Geometry: final body of the model. Coordinates: model frame, mm. Face numbers are marked on the shaded views. A direction names the side the tool comes from. Coordinates: 2 decimals unless noted, no trailing zeros. Loops run counter-clockwise (first coordinate to the right, second up) from the corner with the lowest first, then second, coordinate; pieces in that order, holes last. Notation, with made-up numbers: (-22.5, 82.25) -> (-14.5, 82.25) arc R14 cw to (-14.5, 92.25) -> close; hole circle Ø1 at (57, -33.75). An arc over 180 degrees is marked (long way). One line per item, written item: value. Start each with the question number.
Item 1: Section query A-A on x = 0. Return loops of the section in (y, z).
Item 2: Set-up query: the marked faces 3 and 4. Return all of +Z, -Z, +X, -X, +Y, -Y with unobstructed straight access to the full face (end or side cutting, diameter ignored); none if empty.
Item 3: Mould query, pull axis X, two halves, no side actions, for the marked faces 1 and 2. Classes: +X half, -X half, draft (parallel to the pull), parting line (faces both ways), or undercut.
Item 4: Section query D-D on z = 4.86. Return loops of the section in (x, y).
Item 5: Section query B-B on z = 0. Return loops of the section in (x, y), then the cut area to 3 significant figures.
Item 6: Contact query for a flat-ended pin moving along its axis: pin 1 Ø2.5 at (x, z) = (6, 4.86) entering from -Y. Output: stop coordinate, or through.
Item 7: Section query C-C on y = 0.7. Return loops of the section in (x, z), then the cut area to 3 significant figures.
Item 8: Ray query, probe 1 along Z at (x, y) = (6, 0.65); probe 2 along X at (y, z) = (0.2, 4.86); probe 3 along X at (y, z) = (0.4, -5.5). Return the intervals inside material, ascending. Write a range as from..to.
Autodesk Inventor part; units mm, degrees
ref_plane "YZ Plane" through (0, 0, 0) normal (1, 0, 0) x (0, 1, 0)
ref_plane "XZ Plane" through (0, 0, 0) normal (0, 1, 0) x (-1, 0, 0)
ref_plane "XY Plane" through (0, 0, 0) normal (0, 0, 1) x (1, 0, 0)
sketch "Sketch1" plane through (0, 0, 0) normal (0, 1, 0) x (-1, 0, 0)
  line L0 (-7.5, 6.36) -> (7.5, 6.36)
  line L1 (7.5, 6.36) -> (7.5, -6.36)
  line L2 (7.5, -6.36) -> (-7.5, -6.36)
  line L3 (-7.5, -6.36) -> (-7.5, 6.36)
  line L4 (-7.5, 6.36) -> (7.5, -6.36) construction
  line L5 (7.5, 6.36) -> (-7.5, -6.36) construction
  point P0 (0, 0)
  dimension "d0" = 12.72
  dimension "d1" = 15
extrude "Extrusion1" add sketch "Sketch1" along normal blind 1
sketch "Sketch2" plane through (0, 1, 0) normal (0, 1, 0) x (1, 0, 0)
  circle A0 centre (0, 0) radius 4
  dimension "d4" = 8
extrude "Extrusion2" cut sketch "Sketch2" against normal up to surface (1 mm away)
sketch "Sketch3" plane through (0, 0, 0) normal (0, -1, 0) x (1, 0, 0)
  circle A0 centre (0, 0) radius 4
  circle A1 centre (0, 0) radius 6
  dimension "d7" = 12
  dimension "d8" = 8
extrude "Extrusion3" add sketch "Sketch3" along normal blind 0.46
sketch "Sketch4" plane through (0, 1, 0) normal (0, 1, 0) x (1, 0, 0)
  point P0 (0, 0)
sketch "Sketch5" plane through (0, 1, 0) normal (0, 1, 0) x (1, 0, 0)
  circle A0 centre (-6, -4.86) radius 0.8
  line L0 (-7.5, 6.36) -> (-7.5, -6.36)
  line L1 (-7.5, 0) -> (7.5, 0) construction
  line L2 (7.5, -6.36) -> (7.5, 6.36)
  line L3 (-7.5, -6.36) -> (7.5, -6.36)
  line L4 (0, -6.36) -> (0, 6.36) construction
  line L5 (7.5, 6.36) -> (-7.5, 6.36)
  circle A1 centre (-6, 4.86) radius 0.8
  line L6 (0, 6.36) -> (0, -6.36) construction
  circle A2 centre (6, -4.86) radius 0.8
  circle A3 centre (6, 4.86) radius 0.8
  point P0 (0, 0)
  dimension "d11" = 1.5
  dimension "d12" = 1.6
  dimension "d13" = 1.5
extrude "Extrusion4" cut sketch "Sketch5" against normal up to surface (1 mm away) contours A0 | A1 | A2 | A3
properties part number "PinholeFlexFixture" material "Acetal Resin, Black"
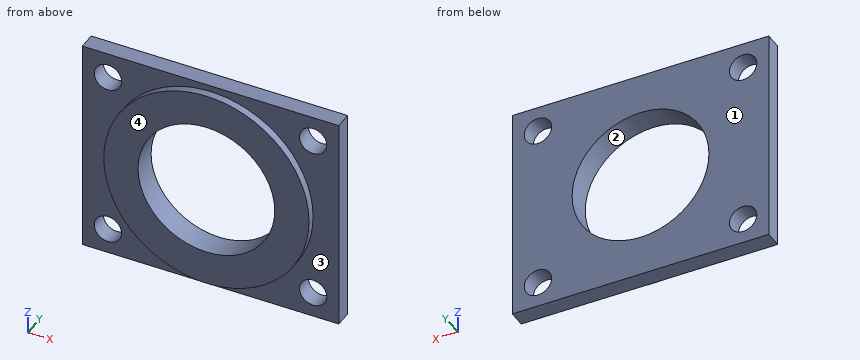
Reply:
1. outline: (-0.46, -6) -> (0, -6) -> (0, -6.36) -> (1, -6.36) -> (1, -4) -> (-0.46, -4) -> close; (-0.46, 4) -> (1, 4) -> (1, 6.36) -> (0, 6.36) -> (0, 6) -> (-0.46, 6) -> close
2. face 3: -Y
2. face 4: +Z, -Z, +X, -X, -Y
3. face 1: draft
3. face 2: undercut
4. outline: (-7.5, 0) -> (-6.8, 0) -> (-6.8, 1) -> (-7.5, 1) -> close; (-5.2, 0) -> (-3.52, 0) -> (-3.52, -0.46) -> (3.52, -0.46) -> (3.52, 0) -> (5.2, 0) -> (5.2, 1) -> (-5.2, 1) -> close; (6.8, 0) -> (7.5, 0) -> (7.5, 1) -> (6.8, 1) -> close
5. outline: (-7.5, 0) -> (-6, 0) -> (-6, -0.46) -> (-4, -0.46) -> (-4, 1) -> (-7.5, 1) -> close; (4, -0.46) -> (6, -0.46) -> (6, 0) -> (7.5, 0) -> (7.5, 1) -> (4, 1) -> close
5. area: 8.84 mm²
6. pin 1: stops at y = 0
7. outline: (-7.5, -6.36) -> (7.5, -6.36) -> (7.5, 6.36) -> (-7.5, 6.36) -> close; hole circle Ø1.6 at (-6, -4.86); hole circle Ø1.6 at (-6, 4.86); hole circle Ø8 at (0, 0); hole circle Ø1.6 at (6, -4.86); hole circle Ø1.6 at (6, 4.86)
7. area: 132 mm²
8. probe 1: z = -6.36..-5.66, -4.06..4.06, 5.66..6.36
8. probe 2: x = -7.5..-6.8, -5.2..5.2, 6.8..7.5
8. probe 3: x = -7.5..-6.48, -5.52..5.52, 6.48..7.5
